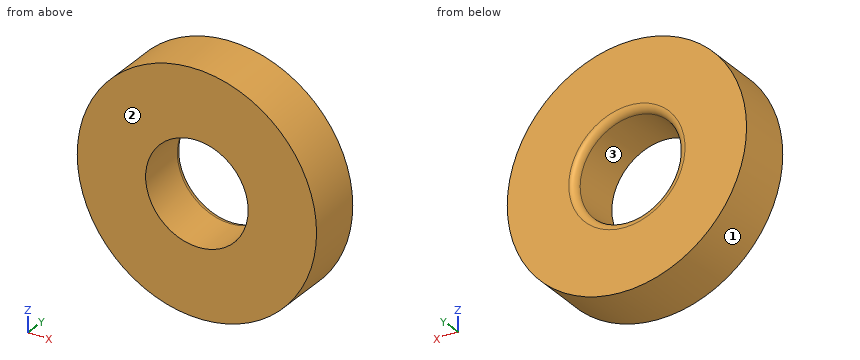
from build123d import *

# Parameters (mm, degrees)
SKETCH1_R           = 17.5
BOSS_EXTRUDE1_DEPTH = 8
SKETCH2_R           = 7.5
CUT_EXTRUDE1_DEPTH  = 9
FILLET1_R           = 1


with BuildPart() as part:
    # Sketch1 → Boss-Extrude1 (new body)
    with BuildSketch(Plane(origin=(0, 0, 0), x_dir=(1, 0, 0), z_dir=(0, 1, 0))):
        Circle(SKETCH1_R)
    extrude(amount=BOSS_EXTRUDE1_DEPTH)

    # Sketch2 → Cut-Extrude1 (cut, through all)
    with BuildSketch(Plane(origin=(0, 8, 0), x_dir=(1, 0, 0), z_dir=(0, 1, 0))):
        Circle(SKETCH2_R)
    extrude(amount=-CUT_EXTRUDE1_DEPTH, mode=Mode.SUBTRACT)

    # Fillet1
    fillet1_edges = [part.edges().sort_by_distance(p)[0] for p in [
        (-7.5, 8, 0),
    ]]
    fillet(fillet1_edges, radius=FILLET1_R)


solid = part.part
Source: CAD feature listing. Evaluate the final solid. Frame: model axes, mm. Face numbers are marked on the shaded views. Give positions to 0.01 mm unless a question says otherwise; leave off trailing zeros. Order: outer loops, then holes, each group sorted by start corner. A loop starts at its lowest first (then second) coordinate and runs counter-clockwise, first axis right, second up. Notation, with made-up numbers: (6, 4.5) -> (30, 4.5) arc R25 ccw to (30, 38.5) -> close; hole circle Ø6 at (18.5, -20). An arc over 180 degrees is marked (long way). Use a Markdown table: item, result.
1) Mould query, pull axis Z, two halves, no side actions, for the marked faces 1, 2 and 3. Classes: +Z half, -Z half, draft (parallel to the pull), parting line (faces both ways), or undercut.
Answer list:
| item | result |
|---|---|
| face 1 | parting line |
| face 2 | draft |
| face 3 | undercut |
2) Contact query for flat-ended pins moving along their axis: P1, Ø3, axis at y = 2.5, z = 9.5, coming from the -X side; P2, Ø2, axis at y = 5.5, z = -1, coming from the +X side; P3, Ø1.5, axis at x = -4.5, y = 5, coming from the -Z side; P4, Ø1, axis at x = 2.5, y = 3, coming from the -Z side. Output: stop coordinate, or through.
Answer list:
| item | result |
|---|---|
| P1 | x = -15.56 |
| P2 | x = 17.5 |
| P3 | z = -17.09 |
| P4 | z = -17.39 |
3) Section query D-D, the plane z = -10.5. Return the cut outline in (x, y), then the cut area to 3 significant figures.
Answer list:
| item | result |
|---|---|
| outline | (-14, 0) -> (14, 0) -> (14, 8) -> (-14, 8) -> close |
| area | 224 mm² |
4) Section query C-C, the plane y = 5.5. Return the cut outline in (x, z).
Answer list:
| item | result |
|---|---|
| outline | circle Ø35 at (0, 0); hole circle Ø15 at (0, 0) |
5) Ray query, line 1 along Z through (x, y) = (0, 2.5); line 2 along Z through (x, y) = (-3.5, 0.5). Return the intervals inside material, ascending. Write a range as [from, to].
Answer list:
| item | result |
|---|---|
| line 1 | [-17.5, -7.5], [7.5, 17.5] |
| line 2 | [-17.15, -6.63], [6.63, 17.15] |
6) Section query A-A, the plane x = 0. Return the cut outline in (y, z), then the cut area to 3 significant figures.
Answer list:
| item | result |
|---|---|
| outline | (0, -17.5) -> (8, -17.5) -> (8, -8.5) arc R1 ccw to (7, -7.5) -> (0, -7.5) -> close; (0, 7.5) -> (7, 7.5) arc R1 ccw to (8, 8.5) -> (8, 17.5) -> (0, 17.5) -> close |
| area | 160 mm² |
7) Section query B-B, the plane z = 0. Return the cut outline in (x, y).
Answer list:
| item | result |
|---|---|
| outline | (-17.5, 0) -> (-7.5, 0) -> (-7.5, 7) arc R1 ccw to (-8.5, 8) -> (-17.5, 8) -> close; (7.5, 0) -> (17.5, 0) -> (17.5, 8) -> (8.5, 8) arc R1 ccw to (7.5, 7) -> close |
